The model under review builds one solid part; all positions refer to its coordinate system, in mm. Face numbers are marked on the shaded views. A direction names the side the tool comes from. Round coordinates to 2 decimals unless told otherwise and drop trailing zeros. Loops run counter-clockwise (first coordinate to the right, second up) from the corner with the lowest first, then second, coordinate; pieces in that order, holes last. Notation, with made-up numbers: M -18,16.25 L 38,16.25 A11 ccw 38,33.25 Z; hole C 40,29.5 d10. An arc over 180 degrees is marked long. Answer as a JSON object with one key per item and string values. Group by question number.
Item 1: The part is to be moulded in two halves that separate along Y. For the marked faces 3, 4 and 5, say which applies: +Y half, -Y half, draft (parallel to the pull), parting line (faces both ways), or undercut.
Item 2: Insertion check: P1, Ø5.5, axis at x = 0, y = 0, coming from the +Z side; P2, Ø1.5, axis at x = -4.5, z = 10, coming from the +Y side; P3, Ø1, axis at x = 0.5, y = -1, coming from the -Z side; P4, Ø3, axis at x = -6, z = 5.5, coming from the +Y side. Each pin has a flat end and moves straight along its axis. Give the tip position at first contact, or say it passes through.
Item 3: To check wall thickness, follow line 1 (X direction, y = 0, z = 7.5); line 2 (Y direction, x = -1.75, z = 0.5); line 3 (X direction, y = 8.25, z = 4.5). State the ranges of each line that lie inside material, in increasing order.
Item 4: Tool access review of the marked faces 1 and 2: name each direction out of +Z, -Z, +X, -X, +Y, -Y from which nothing blocks a thin tool from reaching the whole face with its end or side.
Item 5: Consider section D-D (x = 5.5). Give the boundary of the cut face in (y, z).
Item 6: Consider section B-B (x = -1.25). Give the boundary of the cut face in (y, z).
Item 7: Consider section A-A (y = 0). Give the boundary of the cut face in (x, z), and give its area (3 significant figures).
Item 8: Consider section C-C (z = 8.75). Give the boundary of the cut face in (x, y), and give its area (3 significant figures).
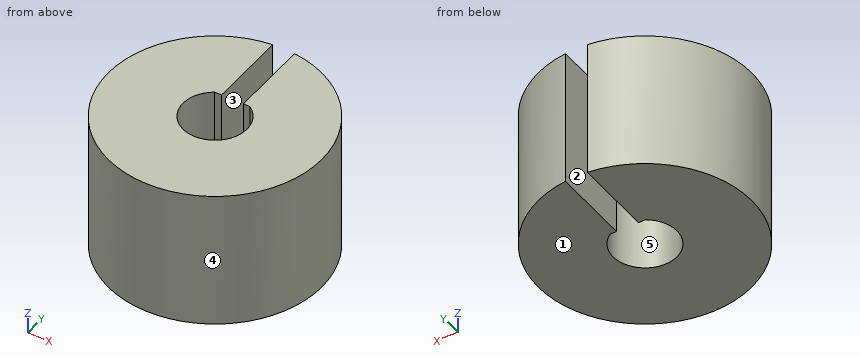
Autodesk Inventor part; units mm, degrees
ref_plane "YZ Plane" through (0, 0, 0) normal (1, 0, 0) x (0, 1, 0)
ref_plane "XZ Plane" through (0, 0, 0) normal (0, 1, 0) x (-1, 0, 0)
ref_plane "XY Plane" through (0, 0, 0) normal (0, 0, 1) x (1, 0, 0)
sketch "Sketch1" plane through (0, 0, 0) normal (0, 0, 1) x (1, 0, 0)
  arc A0 (-1.6583, 2.5) -> (1.6583, 2.5) centre (0, 0) ccw
  arc A1 (-1, 9.9499) -> (1.0526, 9.9444) centre (0, 0) ccw
  line L0 (1.0526, 2.5) -> (1.0526, 9.9444)
  line L1 (-1, 9.9499) -> (-1, 2.5)
  line L2 (-1.6583, 2.5) -> (-1, 2.5)
  line L3 (1.0526, 2.5) -> (1.6583, 2.5)
  dimension "d0" = 6
  dimension "d2" = 20
  dimension "d4" = 1
extrude "Extrusion1" add sketch "Sketch1" along normal blind 13
equation "\"BendRadius\" = Thickness"
equation "\"BendReliefWidth\" = Thickness"
equation "\"BendReliefDepth\" = 0.5 * Thickness"
equation "\"CornerReliefSize\" = 4 * Thickness"
equation "\"MinimumRemnant\" = 2 * Thickness"
equation "\"TransitionRadius\" = BendRadius"
equation "\"JacobiRadiusSize\" = BendRadius"
equation "\"GapSize\" = Thickness"
properties part number "Reducer bushing"
Geometry results:
{
 "1": {"face 3": "draft", "face 4": "parting line", "face 5": "undercut"},
 "2": {"P1": "stops at z = 13", "P2": "stops at y = 9.27", "P3": "passes through", "P4": "stops at y = 8.93"},
 "3": {"line 1": "x = -10 to -3, 3 to 10", "line 2": "y = -9.85 to -2.44, 2.44 to 9.85", "line 3": "x = -5.65 to -1, 1.05 to 5.65"},
 "4": {"face 1": "-Z, +X, -X, +Y, -Y", "face 2": "+Z, -Z, +Y"},
 "5": {"outline": "M -8.35,0 L 8.35,0 L 8.35,13 L -8.35,13 Z"},
 "6": {"outline": "M -9.92,0 L -2.73,0 L -2.73,13 L -9.92,13 Z; M 2.5,0 L 9.92,0 L 9.92,13 L 2.5,13 Z"},
 "7": {"outline": "M -10,0 L -3,0 L -3,13 L -10,13 Z; M 3,0 L 10,0 L 10,13 L 3,13 Z", "area": "182 mm^2"},
 "8": {"outline": "M -1.66,2.5 L -1,2.5 L -1,9.95 A10 ccw long 1.05,9.94 L 1.05,2.5 L 1.66,2.5 A3 cw long Z", "area": "272 mm^2"}
}
